Source: three-view drawing plus pictorial views. Frame: mm from the lowest corner of the part. Coordinates: 2 decimals unless noted, no trailing zeros. Write each loop counter-clockwise with the first axis right and the second up, starting at its lowest first coordinate (ties: lowest second). Pieces come first, ordered by that corner, then holes. Notation, with made-up numbers: (-39, 72) - (-26, 72) arc R22 cw to (-26, 82) - close; hole circle Ø6 at (89, 81). An arc over 180 degrees is marked (long way). One line per item, written item: value.
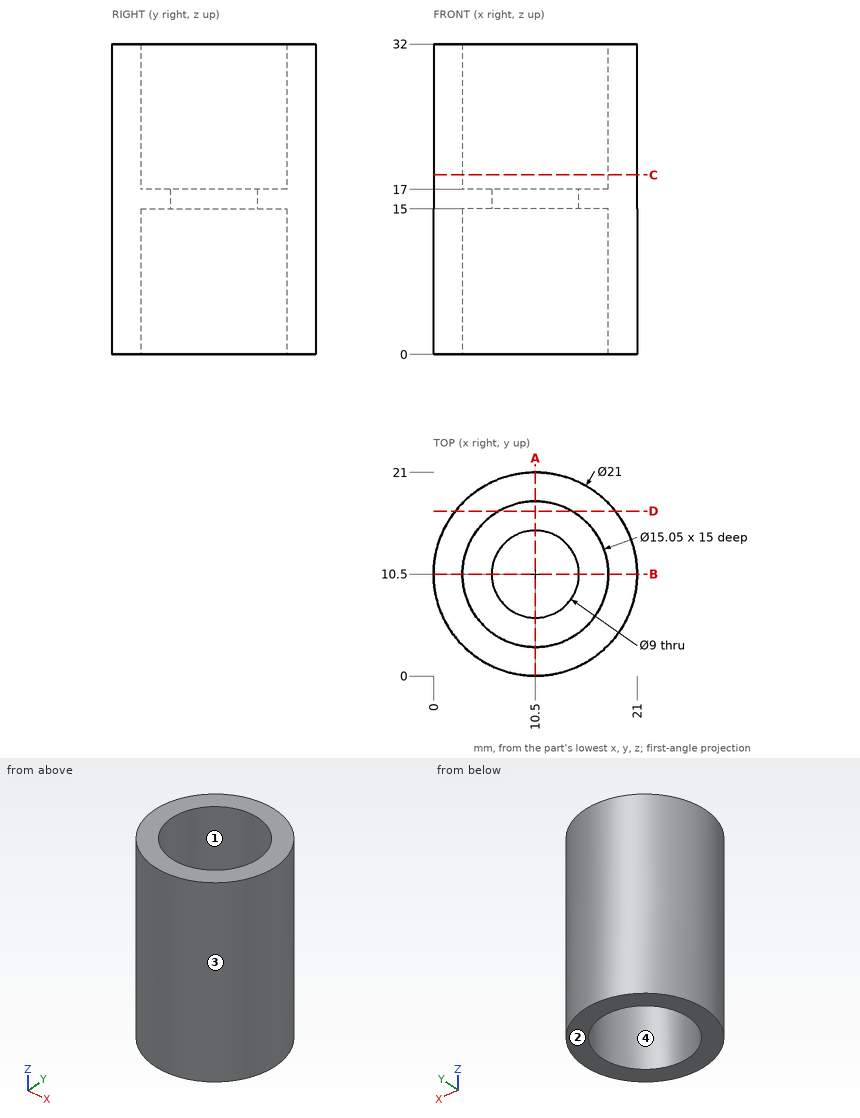
1) Material intervals for line 1 (Y direction, x = 10.5, z = 5.25) (3 decimals); line 2 (Z direction, x = 7, y = 4); line 3 (Y direction, x = 15, z = 25), sorted ascending.
Values found:
line 1: 0 to 2.975, 18.025 to 21
line 2: 15 to 17
line 3: 1.01 to 4.47, 16.53 to 19.99
2) Contact query for flat-ended pins moving along their axis: P1, Ø10.5, axis at x = 10.5, y = 10.5, coming from the +Z side; P2, Ø1, axis at y = 19, z = 28.5, coming from the -X side; P3, Ø3, axis at y = 8.5, z = 12.5, coming from the +X side. Output: stop coordinate, or through.
Values found:
P1: z = 17
P2: x = 3.7
P3: x = 20.99
3) Section query A-A on x = 10.5. Output: boundary loops of the cut face in (y, z) (3 decimals).
Values found:
outline: (0, 0) - (2.975, 0) - (2.975, 15) - (6, 15) - (6, 17) - (2.975, 17) - (2.975, 32) - (0, 32) - close; (15, 15) - (18.025, 15) - (18.025, 0) - (21, 0) - (21, 32) - (18.025, 32) - (18.025, 17) - (15, 17) - close
4) Section query C-C on z = 18.5. Output: boundary loops of the cut face in (x, y) (3 decimals), then the cut area to 3 significant figures.
Values found:
outline: circle Ø21 at (10.5, 10.5); hole circle Ø15.05 at (10.5, 10.5)
area: 168 mm2
5) Section query D-D on y = 17. Output: boundary loops of the cut face in (x, z), then the cut area to 3 significant figures.
Values found:
outline: (2.25, 0) - (6.71, 0) - (6.71, 15) - (14.29, 15) - (14.29, 0) - (18.75, 0) - (18.75, 32) - (14.29, 32) - (14.29, 17) - (6.71, 17) - (6.71, 32) - (2.25, 32) - close
area: 300 mm2
6) Draft query along X for the marked faces 1, 2, 3 and 4. Return one class per face: released by +X, released by -X, zero draft, split by the parting line, or undercut.
Values found:
face 1: undercut
face 2: zero draft
face 3: split by the parting line
face 4: undercut
